from build123d import *

# Parameters (mm, degrees)
ESBO_O1_W                        = 50
ESBO_O1_H                        = 50
RESSALTO_EXTRUS_O1_DEPTH         = 6.35
FURO_COM_FOLGA_DE_M131_D         = 20
FURO_DE_DI_METRO_3_3_3_3_2_D     = 3.3
FURO_DE_DI_METRO_3_3_3_3_2_DEPTH = 9.1
FURO_DE_DI_METRO_3_3_3_3_2_TIP   = 0.991420021
FILETE1_R                        = 9.525


with BuildPart() as part:
    # Esboço1 → Ressalto-extrusão1 (new body)
    with BuildSketch(Plane.XY.offset(6.35)):
        with Locations((12, 25)):
            Rectangle(ESBO_O1_W, ESBO_O1_H)
    extrude(amount=-RESSALTO_EXTRUS_O1_DEPTH)

    # Furo com folga de M131 (through all)
    with Locations(Plane(origin=(0, 0, 0), x_dir=(-1, 0, 0), z_dir=(0, 0, -1))):
        with Locations((-12, 25.5)):
            Hole(FURO_COM_FOLGA_DE_M131_D / 2)

    # Furo de diâmetro Ø3.3 (3.3)2
    with Locations(Plane(origin=(0, 0, 0), x_dir=(-1, 0, 0), z_dir=(0, -1, 0))):
        with Locations((5.5, -3.175), (-29.5, -3.175)):
            Hole(FURO_DE_DI_METRO_3_3_3_3_2_D / 2, depth=FURO_DE_DI_METRO_3_3_3_3_2_DEPTH)
            with Locations((0, 0, -(FURO_DE_DI_METRO_3_3_3_3_2_DEPTH + FURO_DE_DI_METRO_3_3_3_3_2_TIP / 2))):  # 118° drill point
                Cone(0, FURO_DE_DI_METRO_3_3_3_3_2_D / 2, FURO_DE_DI_METRO_3_3_3_3_2_TIP, mode=Mode.SUBTRACT)

    # Filete1
    filete1_edges = [part.edges().sort_by_distance(p)[0] for p in [
        (-13, 50, 3.175),
        (37, 50, 3.175),
    ]]
    fillet(filete1_edges, radius=FILETE1_R)


solid = part.part
The model under review builds one solid part; all positions refer to its coordinate system, in mm. A direction names the side the tool comes from. Round coordinates to 2 decimals unless told otherwise and drop trailing zeros. Loops run counter-clockwise (first coordinate to the right, second up) from the corner with the lowest first, then second, coordinate; pieces in that order, holes last. Notation, with made-up numbers: (44.25, -33.75) -> (64.25, -33.75) arc R25 cw to (64.25, -16.75) -> close; hole circle Ø3 at (-25, 55). An arc over 180 degrees is marked (long way). One line per question, with ' | ' between items. Start each with the question number.
Item 1: For pin 1 (2 mm diameter, centred on y = 44, z = 1, fed in from +X); pin 2 (1.5 mm diameter, centred on x = -7, z = 5, fed in from +Y); pin 3 (3 mm diameter, centred on x = 29.5, z = 3.175, fed in from +Y), all flat-tipped, find the tip position at first contact; note any pin that passes through.
Item 2: Draft analysis for pull direction Z (two halves, no side actions). For faces 1 (the face through (12, 0, 3)), 2 (the face through (-5.44, 9.92, 3.45)), 3 (the face through (12, 14, 0)), state which applies: +Z half, -Z half, draft (parallel to the pull), parting line (faces both ways), or undercut.
Item 3: Wall thickness on line 1 along Y through (x, z) = (11.5, 3.5); line 2 along Z through (x, y) = (-5.5, 3.5) (3 decimals); line 3 along X through (y, z) = (3, 4.25): over which ranges is each line inside the solid? List them lowest first. Write a range as [from, to].
Item 4: Add section B-B, the plane x = 12. Write out the cut boundary in (y, z).
Item 5: Add section C-C, the plane x = 33. Write out the cut boundary in (y, z).
Item 6: Machinability: for faces 4 (the face through (27.85, 4.61, 3.1)), 5 (the face through (-10.28, 47.14, 3.13)), which of the approach directions +Z, -Z, +X, -X, +Y, -Y give a long, thin tool a straight path to every point of the face, cutting with its end or side? Answer none if there is none.
Item 7: Add section A-A, the plane y = 25.5. Write out the cut boundary in (x, z), then the cut area to 4 significant figures.
Return value:
1) pin 1: stops at x = 36.66 | pin 2: stops at y = 49.59 | pin 3: stops at y = 49.99
2) face 1: draft | face 2: undercut | face 3: -Z half
3) line 1: y = [0, 15.51], [35.49, 50] | line 2: z = [0, 1.525], [4.825, 6.35] | line 3: x = [-13, -6.75], [-4.25, 28.25], [30.75, 37]
4) outline: (0, 0) -> (15.5, 0) -> (15.5, 6.35) -> (0, 6.35) -> close; (35.5, 0) -> (50, 0) -> (50, 6.35) -> (35.5, 6.35) -> close
5) outline: (0, 0) -> (48.23, 0) -> (48.23, 6.35) -> (0, 6.35) -> close
6) face 4: -Y | face 5: +Z, -Z, -X, +Y
7) outline: (-13, 0) -> (2, 0) -> (2, 6.35) -> (-13, 6.35) -> close; (22, 0) -> (37, 0) -> (37, 6.35) -> (22, 6.35) -> close | area: 190.5 mm2
